Model file for the job. Use its own axes, mm. A direction names the side the tool comes from. Round coordinates to 2 decimals unless told otherwise and drop trailing zeros. Order: outer loops, then holes, each group sorted by start corner. A loop starts at its lowest first (then second) coordinate and runs counter-clockwise, first axis right, second up. Notation, with made-up numbers: (24.5, 11) - (74.5, 11) arc R8 ccw to (74.5, 15) - close; hole circle Ø5 at (1, 0.25). An arc over 180 degrees is marked (long way). Put each result on its own line as item: value. Start each with the question number.
Item 1: Saw through at D-D on y = 0.3. List the corners of the cut face in (x, z), plus the area to 3 significant figures.
Item 2: Pin check, flat tips, straight feed: pin 1 Ø1.6 at (y, z) = (1.5, 5.5) entering from +X; pin 2 Ø1.6 at (x, y) = (1.5, 1) entering from +Z; pin 3 Ø0.8 at (x, z) = (1, 1.5) entering from +Y. Stop position of each tip, or through.
Item 3: Saw through at B-B on x = -1.25. List the corners of the cut face in (y, z), plus the area to 3 significant figures.
Item 4: Mould opens along Z. For faces 1 (the face through (0, 0, 0)), 2 (the face through (-2, 1, 5)), 3 (the face through (-1.5, 1.5, 4)), 4 (the face through (-1, 0, 8)) say: pulls with the +Z half, pulls with the -Z half, needs draft (parallel to the pull), parting line crosses it, or undercut.
Item 5: Which spindle directions (+Z, -Z, +X, -X, +Y, -Y) get a long thin tool onto all of the face, cutting with end or side? Do faces 5 (the face through (-1.5, -1.5, 4.1)), 6 (the face through (1, 0, 4)), 7 (the face through (-1.5, 1.5, 6)). Say none if no direction does.
Item 6: Probe probe 1 along Z at (x, y) = (-0.85, 1.2); probe 2 along X at (y, z) = (-1.8, 2); probe 3 along Z at (x, y) = (-0.15, 0.5). List the from-to ranges inside material, lowest first.
Item 7: Saw through at A-A on y = 1.3. List the corners of the cut face in (x, z), plus the area to 3 significant figures.
Item 8: Saw through at C-C on z = 2.75. List the corners of the cut face in (x, y).
```python
from build123d import *

# Parameters (mm, degrees)
SKETCH1_W           = 5
SKETCH1_H           = 4
BOSS_EXTRUDE1_DEPTH = 8
SKETCH2_W           = 2
SKETCH2_H           = 2
SKETCH2_H_2         = 1
CUT_EXTRUDE1_DEPTH  = 1
SKETCH4_W           = 6.112752517
SKETCH4_H           = 2
CUT_EXTRUDE2_DEPTH  = 3
SKETCH5_W           = 2
SKETCH5_H           = 3
CUT_EXTRUDE3_DEPTH  = 3
SKETCH6_W           = 3
SKETCH6_H           = 1
CUT_EXTRUDE5_DEPTH  = 9


with BuildPart() as part:
    # Sketch1 → Boss-Extrude1 (new body)
    with BuildSketch(Plane.XY):
        Rectangle(SKETCH1_W, SKETCH1_H)
    extrude(amount=BOSS_EXTRUDE1_DEPTH)

    # Sketch2 → Cut-Extrude1 (cut)
    with BuildSketch(Plane(origin=(0, 2, 0), x_dir=(1, 0, 0), z_dir=(0, 1, 0))):
        with Locations((-1.5, -5)):
            Rectangle(SKETCH2_W, SKETCH2_H)
        with Locations((1.5, -1.5)):
            Rectangle(SKETCH2_W, SKETCH2_H_2)
    extrude(amount=-CUT_EXTRUDE1_DEPTH, mode=Mode.SUBTRACT)

    # Sketch4 → Cut-Extrude2 (cut)
    with BuildSketch(Plane(origin=(2.5, 0, 0), x_dir=(0, 0, -1), z_dir=(1, 0, 0))):
        with Locations((-5.056376259, 1)):
            Rectangle(SKETCH4_W, SKETCH4_H)
    extrude(amount=-CUT_EXTRUDE2_DEPTH, mode=Mode.SUBTRACT)

    # Sketch5 → Cut-Extrude3 (cut)
    with BuildSketch(Plane(origin=(0, 0, 0), x_dir=(1, 0, 0), z_dir=(0, 1, 0))):
        with Locations((1.5, -6.5)):
            Rectangle(SKETCH5_W, SKETCH5_H)
    extrude(amount=-CUT_EXTRUDE3_DEPTH, mode=Mode.SUBTRACT)

    # Sketch6 → Cut-Extrude5 (cut, through all)
    with BuildSketch(Plane.XY.offset(8)):
        with Locations((0, -1.5)):
            Rectangle(SKETCH6_W, SKETCH6_H)
    extrude(amount=-CUT_EXTRUDE5_DEPTH, mode=Mode.SUBTRACT)


solid = part.part
```
Results found:
1. outline: (-2.5, 0) - (2.5, 0) - (2.5, 2) - (-0.5, 2) - (-0.5, 8) - (-2.5, 8) - close
1. area: 22.0 mm²
2. pin 1: stops at x = -0.5
2. pin 2: stops at z = 2
2. pin 3: stops at y = 1
3. outline: (-1, 0) - (2, 0) - (2, 4) - (1, 4) - (1, 6) - (2, 6) - (2, 8) - (-1, 8) - close
3. area: 22.0 mm²
4. face 1: pulls with the -Z half
4. face 2: undercut
4. face 3: undercut
4. face 4: pulls with the +Z half
5. face 5: +Z, -Z, -Y
5. face 6: +Z, +X, +Y
5. face 7: +X, -X, +Y
6. probe 1: z = 0 to 4, 6 to 8
6. probe 2: x = -2.5 to -1.5, 1.5 to 2.5
6. probe 3: z = 0 to 2
7. outline: (-2.5, 0) - (2.5, 0) - (2.5, 1) - (0.5, 1) - (0.5, 2) - (-0.5, 2) - (-0.5, 4) - (-2.5, 4) - close; (-2.5, 6) - (-0.5, 6) - (-0.5, 8) - (-2.5, 8) - close
7. area: 16.0 mm²
8. outline: (-2.5, -2) - (-1.5, -2) - (-1.5, -1) - (1.5, -1) - (1.5, -2) - (2.5, -2) - (2.5, 0) - (-0.5, 0) - (-0.5, 2) - (-2.5, 2) - close
